Here's how the part is built. I have some questions about the finished solid (model axes, mm). Face numbers are marked on the shaded views. A direction names the side the tool comes from. Round coordinates to 2 decimals unless told otherwise and drop trailing zeros. Order: outer loops, then holes, each group sorted by start corner. A loop starts at its lowest first (then second) coordinate and runs counter-clockwise, first axis right, second up. Notation, with made-up numbers: M 8.5,15 L 64.5,15 A24 ccw 64.5,36 Z; hole C 48.5,35.25 d3. An arc over 180 degrees is marked long. Write each question's results on one line, items separated by ' | '. Start each with the question number.
```python
from build123d import *

# Parameters (mm, degrees)
F0_W     = 65
F0_H     = 30
F0_R     = 1.375
F1_DEPTH = 1.6
F2_R     = 3
F3_W     = 12
F3_H     = 12
F4_DEPTH = 2
F5_W     = 11.2
F5_H     = 7
F6_DEPTH = 3
F7_W     = 7.5
F7_H     = 5
F8_DEPTH = 2.5


with BuildPart() as f1:
    # F0 (on Top) → F1 (new body)
    with BuildSketch(Plane.XY):
        Rectangle(F0_W, F0_H)
        with Locations((-29, -11.5)):
            Circle(F0_R, mode=Mode.SUBTRACT)
        with Locations((29, -11.5)):
            Circle(F0_R, mode=Mode.SUBTRACT)
        with Locations((-29, 11.5)):
            Circle(F0_R, mode=Mode.SUBTRACT)
        with Locations((29, 11.5)):
            Circle(F0_R, mode=Mode.SUBTRACT)
    extrude(amount=F1_DEPTH)

    # F2
    f2_edges = [f1.edges().sort_by_distance(p)[0] for p in [
        (-32.5, -15, 0.8),
        (-32.5, 15, 0.8),
        (32.5, -15, 0.8),
        (32.5, 15, 0.8),
    ]]
    fillet(f2_edges, radius=F2_R)

    # F3 (on face) → F4 (join)
    with BuildSketch(Plane.XY.offset(1.6)):
        with Locations((-25, 1.9)):
            Rectangle(F3_W, F3_H)
    extrude(amount=F4_DEPTH)

    # F5 (on face) → F6 (join)
    with BuildSketch(Plane.XY.offset(1.6)):
        with Locations((-20.1, -12.5)):
            Rectangle(F5_W, F5_H)
    extrude(amount=F6_DEPTH)

    # F7 (on face) → F8 (join)
    with BuildSketch(Plane.XY.offset(1.6)):
        with Locations((8.9, -13.5)):
            Rectangle(F7_W, F7_H)
        with Locations((21.5, -13.5)):
            Rectangle(F7_W, F7_H)
    extrude(amount=F8_DEPTH)


solid = f1.part
```
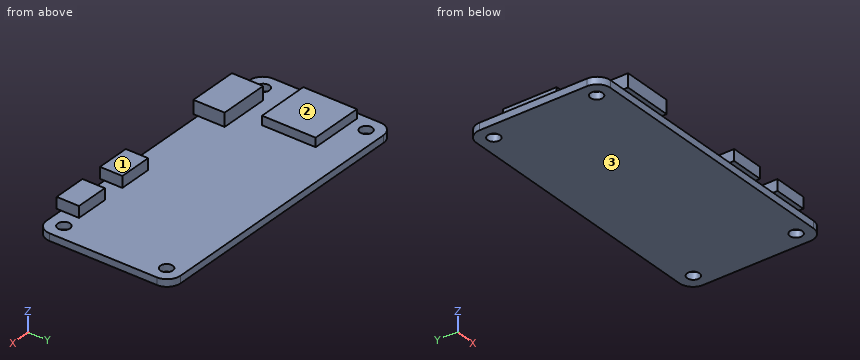
(1) Please list where these lines run through material, in increasing order: line 1 (Y direction, x = -29, z = 0.5) (3 decimals); line 2 (Y direction, x = 7, z = 2.6); line 3 (Z direction, x = 27, y = -13).
(2) I want a section at B-B on y = -3. Write out the boundary of the cut face in (x, z), and give its area (3 significant figures).
(3) I want a section at C-C on x = -26.5. Write out the boundary of the cut face in (y, z).
(4) On a 3-axis mill with a long thin cutter (end or side, diameter ignored), from which of +Z, -Z, +X, -X, +Y, -Y can I reach the whole of each face in a straight line? I mean the marked faces 1, 2 and 3. Say none if no direction works.
(5) I'm going to push flat-ended pins straight in: pin 1 Ø4 at (x, y) = (9.5, -12.5) entering from +Z; pin 2 Ø1.2 at (y, z) = (-13, 2.5) entering from -X; pin 3 Ø0.5 at (x, z) = (4.5, 0.5) entering from -Y. Where does each tip first touch, or does it pass through?
(6) I want a section at A-A on z = 2.6. Write out the boundary of the cut face in (x, y), and give its area (3 significant figures).
(7) I want a section at D-D on x = 26. Write out the boundary of the cut face in (y, z), and give its area (3 significant figures).
Solutions:
1) line 1: -15 to -12.875, -10.125 to 10.125, 12.875 to 15 | line 2: -16 to -11 | line 3: 0 to 1.6
2) outline: M -32.5,0 L 32.5,0 L 32.5,1.6 L -19,1.6 L -19,3.6 L -31,3.6 L -31,1.6 L -32.5,1.6 Z | area: 128 mm^2
3) outline: M -15,0 L 15,0 L 15,1.6 L 7.9,1.6 L 7.9,3.6 L -4.1,3.6 L -4.1,1.6 L -15,1.6 Z
4) face 1: +Z, +X, +Y, -Y | face 2: +Z, +X, -X, +Y | face 3: -Z, +X, -X, +Y, -Y
5) pin 1: z = 4.1 | pin 2: x = -25.7 | pin 3: y = -15
6) outline: M -31,-4.1 L -19,-4.1 L -19,7.9 L -31,7.9 Z; M -25.7,-16 L -14.5,-16 L -14.5,-9 L -25.7,-9 Z; M 5.15,-16 L 12.65,-16 L 12.65,-11 L 5.15,-11 Z; M 17.75,-16 L 25.25,-16 L 25.25,-11 L 17.75,-11 Z | area: 297 mm^2
7) outline: M -15,0 L 15,0 L 15,1.6 L -15,1.6 Z | area: 48.0 mm^2
